Check sheet for the drawn part. Datum: minimum x, y, z corner. Units: mm. A direction names the side the tool comes from. Coordinates: 2 decimals unless noted, no trailing zeros. Write each loop counter-clockwise with the first axis right and the second up, starting at its lowest first coordinate (ties: lowest second). Pieces come first, ordered by that corner, then holes. Notation, with made-up numbers: (45.25, 45.5) -> (74.25, 45.5) arc R26 cw to (74.25, 66.5) -> close; hole circle Ø2 at (29, 77.5). An arc over 180 degrees is marked (long way). Write item = value, one per line. Start each with the question number.
(1) Section check B-B (y = 3.55). Record the cut outline in (x, z), plus the area to 3 significant figures.
(2) Section check C-C (x = 1.5). Record the cut outline in (y, z).
(3) Section check D-D (y = 5.4). Record the cut outline in (x, z).
(4) Section check A-A (z = 6.5). Record the cut outline in (x, y).
(5) Set-up check for the marked faces 4 and 5: record each of +Z, -Z, +X, -X, +Y, -Y from which the full face is reachable in a straight line by a thin tool's end or side.
(6) Mould release check, pull along Z, two halves, no side actions. Record for the marked faces 1, 2 and 3: released by +Z, released by -Z, zero draft, split by the parting line, or undercut.
(7) Gauge pin test, flat end, axial feed: pin 1 Ø7.5 at (x, z) = (13.5, 10.5) entering from +Y. Record the tip position at first contact, or that the pin passes through.
(8) Material ranges on probe 1 along X at (y, z) = (1.85, 12.5); probe 2 along X at (y, z) = (3.1, 12.5), recorded low to high. Write a range as [from, to].
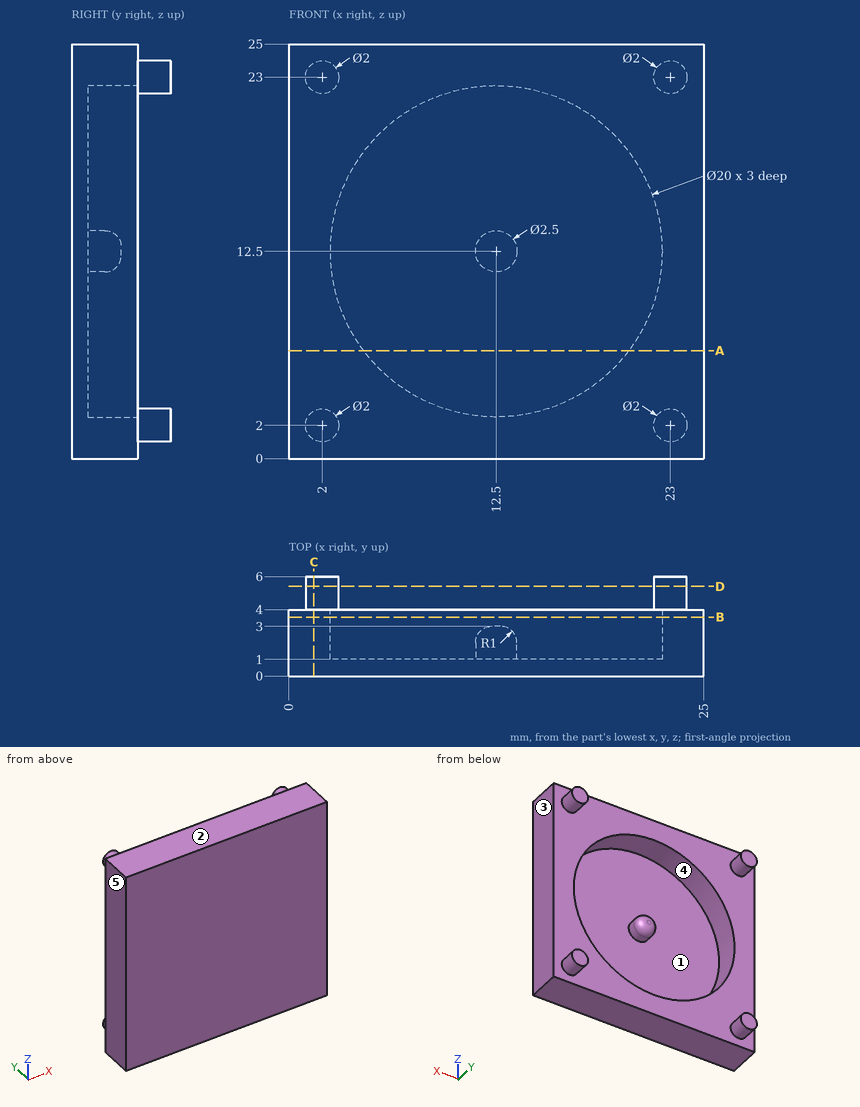
Response:
q1.outline = (0, 0) -> (25, 0) -> (25, 25) -> (0, 25) -> close; hole circle Ø20 at (12.5, 12.5)
q1.area = 311 mm2
q2.outline = (0, 0) -> (4, 0) -> (4, 1.13) -> (6, 1.13) -> (6, 2.87) -> (4, 2.87) -> (4, 22.13) -> (6, 22.13) -> (6, 23.87) -> (4, 23.87) -> (4, 25) -> (0, 25) -> close
q3.outline = circle Ø2 at (2, 2); circle Ø2 at (2, 23); circle Ø2 at (23, 2); circle Ø2 at (23, 23)
q4.outline = (0, 0) -> (25, 0) -> (25, 4) -> (20.5, 4) -> (20.5, 1) -> (4.5, 1) -> (4.5, 4) -> (0, 4) -> close
q5.face_4 = +Y
q5.face_5 = +Z, -Z, -X, +Y, -Y
q6.face_1 = undercut
q6.face_2 = released by +Z
q6.face_3 = zero draft
q7.pin_1 = 3
q8.probe_1 = [0, 2.5], [11.25, 13.75], [22.5, 25]
q8.probe_2 = [0, 2.5], [22.5, 25]
